```python
from build123d import *

# Parameters (mm, degrees)
F1_DEPTH = 63.5
F0_W     = 25.4
F0_H     = 19.05
F2_DEPTH = 25.4
F3_DEPTH = 7.9375
F0_H_2   = 7.599701224
F0_H_3   = 1.925298776
F5_R     = 6.35


with BuildPart() as f1:
    # F0 (on Front) → F1 (new body, symmetric)
    with BuildSketch(Plane.XZ):
        Polygon((-41.275, 9.525), (-41.275, -9.525), (41.275, -9.525), (41.275, 9.525), (22.225, 9.525), align=None)
    extrude(amount=F1_DEPTH, both=True)

    # F0 (on Front) → F2 (join, symmetric)
    with BuildSketch(Plane.XZ):
        with BuildLine():
            Line((22.225, 9.525), (41.275, 9.525))
            Line((41.275, 9.525), (41.275, 33.0692907344))
            ThreePointArc((41.275, 33.0692907344), (45.7386926547, 43.8455980797), (56.515, 48.3092907344))
            Line((56.515, 48.3092907344), (67.8493125877, 48.3092907344))
            Line((67.8493125877, 48.3092907344), (67.8493125877, 67.3592907344))
            Line((67.8493125877, 67.3592907344), (56.515, 67.3592907344))
            ThreePointArc((56.515, 67.3592907344), (32.2683084731, 57.3159822613), (22.225, 33.0692907344))
            Line((22.225, 33.0692907344), (22.225, 9.525))
        make_face()
        with Locations((80.5493125877, 57.8342907344)):
            Rectangle(F0_W, F0_H)
    extrude(amount=F2_DEPTH, both=True)

    # F0 (on Front) → F3 (join, symmetric)
    with BuildSketch(Plane.XZ):
        with BuildLine():
            add(Edge.make_bspline(
                [(-41.275, 9.525), (-22.9515824467, 59.1003261507), (14.3447369337, 68.8547492027), (56.515, 67.3592907344)],
                knots=[0, 0, 0, 0, 113.6120120619, 113.6120120619, 113.6120120619, 113.6120120619], degree=3))
            Line((-41.275, 9.525), (22.225, 9.525))
            Line((22.225, 9.525), (22.225, 33.0692907344))
            ThreePointArc((22.225, 33.0692907344), (32.2683084731, 57.3159822613), (56.515, 67.3592907344))
        make_face()
    extrude(amount=F3_DEPTH, both=True)

    # F0 (on Front) → F4 (revolve)
    with BuildSketch(Plane.XZ):
        with Locations((105.9493125877, 44.5094401224)):
            Rectangle(F0_W, F0_H_2)
        with Locations((105.9493125877, 57.8342907344)):
            Rectangle(F0_W, F0_H)
        with Locations((105.9493125877, 68.3219401224)):
            Rectangle(F0_W, F0_H_3)
    revolve(axis=Axis((93.2493125877, 0, 54.9970895104), (0, 0, 1)))

    # F5
    f5_edges = [f1.edges().sort_by_distance(p)[0] for p in [
        (-41.275, -63.5, 0),
        (41.275, -63.5, 0),
        (41.275, 63.5, 0),
        (-41.275, 63.5, 0),
    ]]
    fillet(f5_edges, radius=F5_R)


solid = f1.part
```
Read the model definition and answer for the solid it produces. Units are mm, in the model's axes. A direction names the side the tool comes from. Give positions to 0.01 mm unless a question says otherwise; leave off trailing zeros. Write each loop counter-clockwise with the first axis right and the second up, starting at its lowest first coordinate (ties: lowest second). Pieces come first, ordered by that corner, then holes. Notation, with made-up numbers: M -28,31.25 L 8,31.25 A31 ccw 8,65.25 Z; hole C -5.5,63.25 d7. An arc over 180 degrees is marked long. Put each result on its own line as item: value. Start each with the question number.
1. The part is cut by section B-B, the plane y = -16.5. Give the vertices of the cut face in (x, z) (3 decimals), and give its area (3 significant figures).
2. For a pull along X with two mould halves and no side action, classify faces 5 (the cylindrical face through (32.536, 16.547, 57.581)), 6 (the flat face through (0, 63.5, 0)), 7 (the cylindrical face through (45.621, -0.356, 43.726)), 8 (the cylindrical face through (117.476, 7.629, 55.197)) as released by +X, released by -X, zero draft, split by the parting line, or undercut.
3. Consider line 1 along Y through (x, z) = (23, 38); line 2 along Y through (x, z) = (19.5, 16); line 3 along X through (y, z) = (-1.5, 6.5) (3 decimals). Determine where each line is inside the solid, lowest interval first.
4. Each of these flat-tipped pins is pushed along its axis until it touches: pin 1 Ø14 at (y, z) = (17.5, 25.5) entering from -X (3 decimals); pin 2 Ø1.5 at (x, z) = (-3.5, 47) entering from +Y; pin 3 Ø18.5 at (x, y) = (72.5, 12) entering from -Z; pin 4 Ø6 at (y, z) = (-40, 13.5) entering from -X. Where does it stop, or does it pass through?
5. The part is cut by section A-A, the plane z = 1.5. Give the vertices of the cut face in (x, y) (3 decimals).
6. Which of the six approach directions +Z, -Z, +X, -X, +Y, -Y give full straight-line access (tool end or side, diameter ignored) to faces 1 (the flat face through (22.225, 17, 21)), 2 (the flat face through (49, -25.4, 52)), 3 (the flat face through (94, 0, 40.71)), 4 (the cylindrical face through (32.536, -16.791, 57.581))?
7. The part is cut by section D-D, the plane y = -52.5. Give the vertices of the cut face in (x, z) (3 decimals), and give its area (3 significant figures).
8. The part is cut by section C-C, the plane y = 20. Give the vertices of the cut face in (x, z) (3 decimals).
Final values:
1. outline: M -41.275,-9.525 L 41.275,-9.525 L 41.275,33.069 A15.24 cw 56.515,48.309 L 73.938,48.309 L 73.938,40.71 L 112.56,40.71 L 112.56,69.285 L 73.938,69.285 L 73.938,67.359 L 56.515,67.359 A34.29 ccw 22.225,33.069 L 22.225,9.525 L -41.275,9.525 Z
1. area: 4,200 mm²
2. face 5: released by -X
2. face 6: zero draft
2. face 7: undercut
2. face 8: undercut
3. line 1: y = -25.4 to 25.4
3. line 2: y = -7.94 to 7.94
3. line 3: x = -41.275 to 41.275
4. pin 1: stops at x = 22.225
4. pin 2: stops at y = 7.94
4. pin 3: stops at z = 40.71
4. pin 4: passes through
5. outline: M -41.275,-57.15 A6.35 ccw -34.925,-63.5 L 34.925,-63.5 A6.35 ccw 41.275,-57.15 L 41.275,57.15 A6.35 ccw 34.925,63.5 L -34.925,63.5 A6.35 ccw -41.275,57.15 Z
6. face 1: +Z, -X, +Y
6. face 2: +Z, +X, -X, -Y
6. face 3: -Z, +X, +Y, -Y
6. face 4: +Z, -X, -Y
7. outline: M -41.275,-9.525 L 41.275,-9.525 L 41.275,9.525 L -41.275,9.525 Z
7. area: 1,570 mm²
8. outline: M -41.275,-9.525 L 41.275,-9.525 L 41.275,33.069 A15.24 cw 56.515,48.309 L 77.592,48.309 L 77.592,40.71 L 108.907,40.71 L 108.907,69.285 L 77.592,69.285 L 77.592,67.359 L 56.515,67.359 A34.29 ccw 22.225,33.069 L 22.225,9.525 L -41.275,9.525 Z
